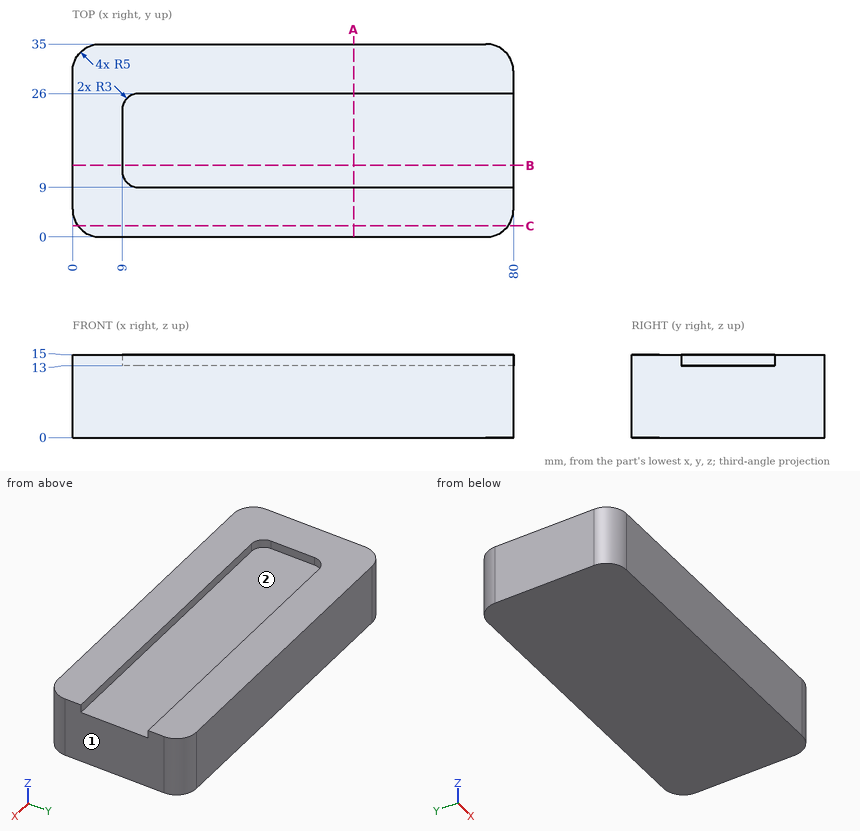
Can you work these out from the drawing? Everything is in mm from the part's minimum corner. A direction names the side the tool comes from. Coordinates: 2 decimals unless noted, no trailing zeros. Write each loop counter-clockwise with the first axis right and the second up, starting at its lowest first coordinate (ties: lowest second). Pieces come first, ordered by that corner, then holes. Notation, with made-up numbers: (29, 70) -> (81, 70) arc R29 cw to (81, 107) -> close; hole circle Ø8 at (-27, 74.25). An arc over 180 degrees is marked (long way). Return JSON: item names as keys, results as strings.
(1) Imagine slicing it at C-C, the plane y = 2. Please give me the cut outline in (x, z).
Numbers:
{"outline": "(1, 0) -> (79, 0) -> (79, 15) -> (1, 15) -> close"}
(2) Which directions (+Z, -Z, +X, -X, +Y, -Y) give clear straight access to the entire face, cutting with the end or side of a thin tool? Please do the marked faces 1 and 2.
Numbers:
{"face 1": "+Z, -Z, +X, +Y, -Y", "face 2": "+Z, +X"}
(3) Imagine slicing it at B-B, the plane y = 13. Please give me the cut outline in (x, z).
Numbers:
{"outline": "(0, 0) -> (80, 0) -> (80, 13) -> (9, 13) -> (9, 15) -> (0, 15) -> close"}
(4) I'm going to push flat-ended pins straight in: pin 1 (1.6 mm diameter, centred on y = 18, z = 14, fed in from +X); pin 2 (8.5 mm diameter, centred on x = 43, y = 19, fed in from +Z). Where does each tip first touch, or does it pass through?
Numbers:
{"pin 1": "stops at x = 9", "pin 2": "stops at z = 13"}
(5) Imagine slicing it at A-A, the plane x = 51. Please give me the cut outline in (y, z).
Numbers:
{"outline": "(0, 0) -> (35, 0) -> (35, 15) -> (26, 15) -> (26, 13) -> (9, 13) -> (9, 15) -> (0, 15) -> close"}
(6) I need wall thicknesses on L1, parallel to Z at x = 42, y = 15; L2, parallel to X at y = 22, z = 13.25; L3, parallel to X at y = 30.5, z = 5.25. Which ranges of each line are inside material? Lowest first, please.
Numbers:
{"L1": "z = 0 to 13", "L2": "x = 0 to 9", "L3": "x = 0.03 to 79.97"}
